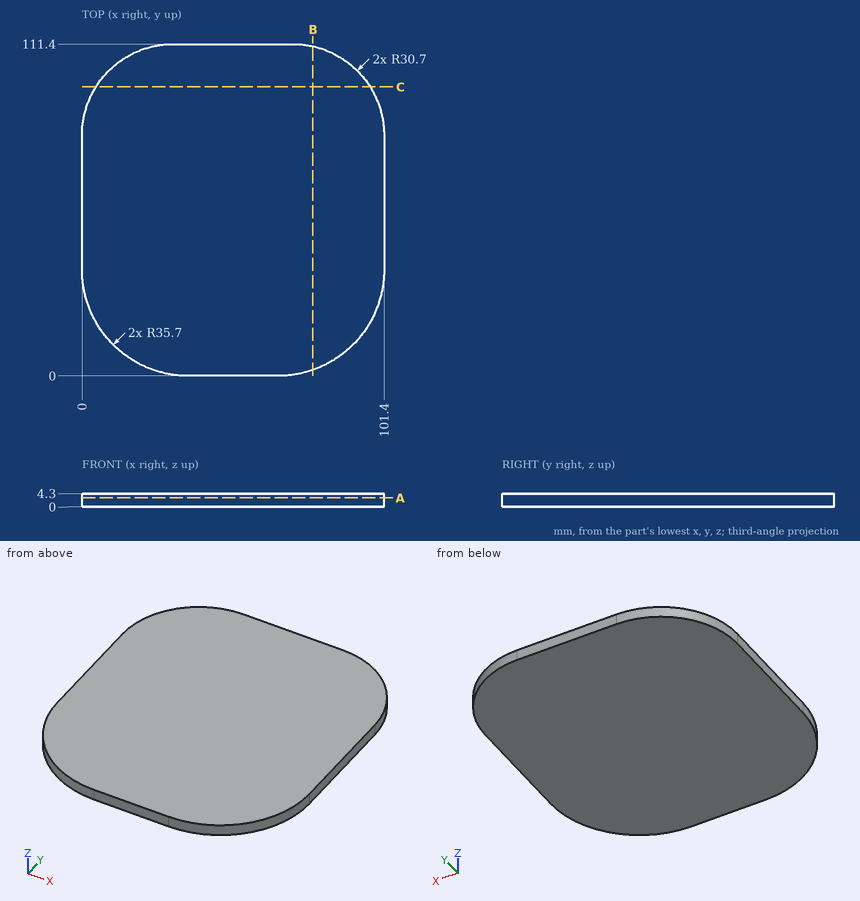
Geometry check sheet. Reference: drawing and pictorial views, mm from the part's lowest x, y, z. Give positions to 0.01 mm unless a question says otherwise; leave off trailing zeros. Loops run counter-clockwise (first coordinate to the right, second up) from the corner with the lowest first, then second, coordinate; pieces in that order, holes last. Notation, with made-up numbers: M -38.5,27.5 L -33.5,27.5 A21 ccw -33.5,43.5 Z; hole C 43.25,54 d1. An arc over 180 degrees is marked long. Use a Markdown table: item, result. Add a question column.
Q1. Sectioned sample at B-B, the plane x = 77.5. Record the cut outline in (y, z), then the cut area to 3 significant figures.
Q2. Scan lines: line 1 along Y through (x, z) = (67, 0.4); line 2 along X through (y, z) = (81.5, 2.25); line 3 along Y through (x, z) = (87.5, 3.5). Record each from-to range of solid material in increasing order. Write a range as [from, to].
Q3. Sectioned sample at A-A, the plane z = 2.95. Record the cut outline in (x, y), then the cut area to 3 significant figures.
Q4. Sectioned sample at C-C, the plane y = 97. Record the cut outline in (x, z).
Verdict:
| question | item | result |
|---|---|---|
| 1 | outline | M 2.01,0 L 110.64,0 L 110.64,4.3 L 2.01,4.3 Z |
| 1 | area | 467 mm^2 |
| 2 | line 1 | [0.02, 111.4] |
| 2 | line 2 | [0.01, 101.39] |
| 2 | line 3 | [7.43, 106.4] |
| 3 | outline | M 0,35.7 A35.7 ccw 35.7,0 L 65.7,0 A35.7 ccw 101.4,35.7 L 101.4,80.7 A30.7 ccw 70.7,111.4 L 30.7,111.4 A30.7 ccw 0,80.7 Z |
| 3 | area | 10,300 mm^2 |
| 4 | outline | M 4.68,0 L 96.72,0 L 96.72,4.3 L 4.68,4.3 Z |
